Autodesk Fusion 360 part; units mm, degrees
sketch "Sketch3" plane through (0, 0, 0) normal (0, 1, 0) x (1, 0, 0)
  circle A0 centre (0, 0) radius 33
  circle A1 centre (0, 0) radius 31
  line L0 (0, 0) -> (0, -31)
  line L1 (0, 0) -> (26.8468, -15.5)
  line L2 (0, 0) -> (31, 0) construction
  circle A2 centre (0, 0) radius 4
  dimension "d8" = 66
  dimension "d9" = 62
  dimension "d10" = 30
  dimension "d11" = 8
extrude "Extrude3" add sketch "Sketch3" along normal blind 4 contours A0 | A1 L0 L1 A2 | L0 L1 A2 | L0 L1 A2 picked at (-10.729, -19.1384)
sketch "Sketch4" plane through (0, 4, 0) normal (0, 1, 0) x (-1, 0, 0)
  arc A0 (0, 31) -> (-26.8468, 15.5) centre (0, 0) ccw
  line L0 (0, 31) -> (0, 4)
  arc A1 (0, 4) -> (-3.4641, 2) centre (0, 0) ccw
  line L1 (-3.4641, 2) -> (-26.8468, 15.5)
  circle A2 centre (0, 0) radius 33
  circle A3 centre (0, 0) radius 2
  circle A4 centre (0, 0) radius 4
  dimension "d14" = 4
  dimension "d15" = 8
extrude "Extrude4" add sketch "Sketch4" along normal blind 2 contours A1 A4
extrude "Extrude5" cut 1 faces at (-0.2436, 4, -0.2863) along direction (0, -1, 0) blind 2
Could you check a few things on this model? Use its own coordinates, in mm. A direction names the side the tool comes from. Round coordinates to 2 decimals unless told otherwise and drop trailing zeros. Write each loop counter-clockwise with the first axis right and the second up, starting at its lowest first coordinate (ties: lowest second). Pieces come first, ordered by that corner, then holes. Notation, with made-up numbers: M -33.5,8.5 L -6.5,8.5 A15 cw -6.5,34.5 Z; hole C 76.25,88.5 d4. An arc over 180 degrees is marked long. Answer in a Markdown table with one row per item. Add a question column.
Q1. If I drill on line 1 (Y direction, x = -26, z = -16.5); line 2 (X direction, y = 0.95, z = 28.5); line 3 (Z direction, x = -4, y = 1.8), over which ranges is the centre line in solid material (lowest first)? Write a range as from..to.
Q2. Imagine slicing it at A-A (z = 0). Please give me the cut outline in (x, y), then the cut area to 3 significant figures.
Q3. Imagine slicing it at C-C (y = 1.25). Please give me the cut outline in (x, z).
Q4. Imagine slicing it at D-D (z = 19.5). Please give me the cut outline in (x, y).
Q5. Imagine slicing it at B-B (x = 14.5). Please give me the cut outline in (y, z), then the cut area to 3 significant figures.
Q6. Will these pins go through, and if not, where does the flat tip stop? pin 1 Ø3 at (x, y) = (-23, 3) entering from -Z (3 decimals); pin 2 Ø2 at (x, z) = (17.5, 22.5) entering from +Y; pin 3 Ø2.5 at (x, z) = (0, 0) entering from +Y; pin 4 Ø1 at (x, y) = (8.5, 2.5) entering from +Z.
Q7. On a 3-axis mill with a long thin cutter (end or side, diameter ignored), from which of +Z, -Z, +X, -X, +Y, -Y can I reach the whole of each face in a straight line? I mean faces 1 (the cylindrical face through (0, 4, 2)), 2 (the flat face through (14.992, 1.972, 8.655)), 3 (the flat face through (0, 0, 0)). Say none if no direction works.
Q8. If we mould it in two halves opening along Z, with no side actions, what happens to faces 4 (the flat face through (2, 6, -1)), 5 (the cylindrical face through (15.7, 1.97, 26.73)), 6 (the cylindrical face through (30.5, 2, -12.6))? For each: +Z half, -Z half, draft (parallel to the pull), parting line (faces both ways), or undercut.
Values:
| question | item | result |
|---|---|---|
| 1 | line 1 | 0..4 |
| 1 | line 2 | -16.64..0, 12.2..16.64 |
| 1 | line 3 | -32.76..32.76 |
| 2 | outline | M -33,0 L 33,0 L 33,4 L 4,4 L 4,6 L 2,6 L 2,2 L -2,2 L -2,6 L -4,6 L -4,4 L -33,4 Z |
| 2 | area | 264 mm^2 |
| 3 | outline | C 0,0 d66; hole M 0,4 A4 cw 3.46,2 L 26.85,15.5 A31 ccw 0,31 Z |
| 4 | outline | M -26.62,0 L 0,0 L 0,4 L -26.62,4 Z; M 24.1,0 L 26.62,0 L 26.62,4 L 24.1,4 Z |
| 5 | outline | M 0,-29.64 L 4,-29.64 L 4,8.37 L 0,8.37 Z; M 0,27.4 L 4,27.4 L 4,29.64 L 0,29.64 Z |
| 5 | area | 161 mm^2 |
| 6 | pin 1 | z = -25.035 |
| 6 | pin 2 | through |
| 6 | pin 3 | y = 2 |
| 6 | pin 4 | z = 32.02 |
| 7 | face 1 | +Y |
| 7 | face 2 | +Y, -Y |
| 7 | face 3 | +Z, -Z, +X, -X, -Y |
| 8 | face 4 | draft |
| 8 | face 5 | undercut |
| 8 | face 6 | parting line |
